Design review of the part shown in the three views and the two pictorial views. Dimensions are in mm from the part's minimum x, y and z. Round coordinates to 2 decimals unless told otherwise and drop trailing zeros. Order: outer loops, then holes, each group sorted by start corner. A loop starts at its lowest first (then second) coordinate and runs counter-clockwise, first axis right, second up.
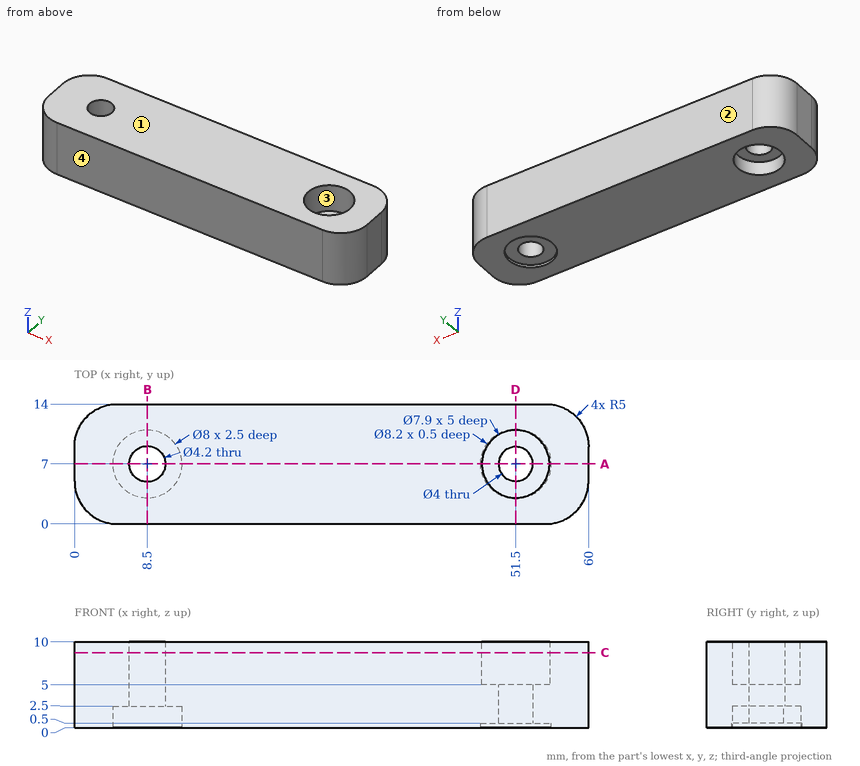
1) Clearance check with flat-ended pins moving along their axes: P1, Ø5, axis at x = 51.5, y = 7, coming from the +Z side; P2, Ø5, axis at x = 8.5, y = 7, coming from the -Z side; P3, Ø2.5, axis at x = 50.5, y = 7, coming from the -Z side. State where each tip first meets the part, or that it passes through.
Results:
P1: stops at z = 5
P2: stops at z = 2.5
P3: stops at z = 0.5
2) Take a section at B-B on x = 8.5. Give the boundary of the cut face in (y, z).
Results:
outline: (0, 0) - (3, 0) - (3, 2.5) - (4.9, 2.5) - (4.9, 10) - (0, 10) - close; (9.1, 2.5) - (11, 2.5) - (11, 0) - (14, 0) - (14, 10) - (9.1, 10) - close
3) Take a section at C-C on z = 8.75. Give the boundary of the cut face in (x, y).
Results:
outline: (0, 5) arc R5 ccw to (5, 0) - (55, 0) arc R5 ccw to (60, 5) - (60, 9) arc R5 ccw to (55, 14) - (5, 14) arc R5 ccw to (0, 9) - close; hole circle Ø4.2 at (8.5, 7); hole circle Ø7.9 at (51.5, 7)
4) The part is to be moulded in two halves that separate along Y. For the marked faces 1, 2, 3 and 4, say which applies: released by +Y, released by -Y, zero draft, split by the parting line, or undercut.
Results:
face 1: zero draft
face 2: released by +Y
face 3: undercut
face 4: released by -Y
5) Take a section at D-D on x = 51.5. Give the boundary of the cut face in (y, z), plus the area to 3 significant figures.
Results:
outline: (0, 0) - (2.9, 0) - (2.9, 0.5) - (5, 0.5) - (5, 5) - (3.05, 5) - (3.05, 10) - (0, 10) - close; (9, 0.5) - (11.1, 0.5) - (11.1, 0) - (14, 0) - (14, 10) - (10.95, 10) - (10.95, 5) - (9, 5) - close
area: 78.4 mm2
6) Take a section at A-A on y = 7. Give the boundary of the cut face in (x, z).
Results:
outline: (0, 0) - (4.5, 0) - (4.5, 2.5) - (6.4, 2.5) - (6.4, 10) - (0, 10) - close; (10.6, 2.5) - (12.5, 2.5) - (12.5, 0) - (47.4, 0) - (47.4, 0.5) - (49.5, 0.5) - (49.5, 5) - (47.55, 5) - (47.55, 10) - (10.6, 10) - close; (53.5, 0.5) - (55.6, 0.5) - (55.6, 0) - (60, 0) - (60, 10) - (55.45, 10) - (55.45, 5) - (53.5, 5) - close
7) To check wall thickness, follow line 1 along Y through (x, z) = (8.5, 8.25); line 2 along Y through (x, z) = (51.5, 7); line 3 along X through (y, z) = (8.75, 6.25). State the ranges of each line that lie inside material, in increasing order.
Results:
line 1: y = 0 to 4.9, 9.1 to 14
line 2: y = 0 to 3.05, 10.95 to 14
line 3: x = 0 to 7.34, 9.66 to 47.96, 55.04 to 60
